```python
from build123d import *

# Parameters (mm, degrees)
SKETCH1_R           = 10
BOSS_EXTRUDE1_DEPTH = 10
FILLET1_R           = 1.5
SKETCH2_R           = 3
CUT_EXTRUDE1_DEPTH  = 8
CHAMFER1_SIZE       = 1


with BuildPart() as part:
    # Sketch1 → Boss-Extrude1 (new body)
    with BuildSketch(Plane.XY):
        Circle(SKETCH1_R)
    extrude(amount=BOSS_EXTRUDE1_DEPTH)

    # Fillet1
    fillet1_edges = [part.edges().sort_by_distance(p)[0] for p in [
        (-10, 0, 0),
        (-10, 0, 10),
    ]]
    fillet(fillet1_edges, radius=FILLET1_R)

    # Sketch2 → Cut-Extrude1 (cut)
    with BuildSketch(Plane(origin=(0, 0, 0), x_dir=(-1, 0, 0), z_dir=(0, 0, -1))):
        Circle(SKETCH2_R)
    extrude(amount=-CUT_EXTRUDE1_DEPTH, mode=Mode.SUBTRACT)

    # Chamfer1
    chamfer1_edges = [part.edges().sort_by_distance(p)[0] for p in [
        (3, 0, 0),
    ]]
    chamfer(chamfer1_edges, length=CHAMFER1_SIZE)

    # Sketch3 → Cut-Revolve2 (revolve, cut)
    with BuildSketch(Plane(origin=(0, 0, 0), x_dir=(0, 0, -1), z_dir=(1, 0, 0))):
        with BuildLine():
            Line((-19, -5), (-9, -5))
            ThreePointArc((-9, -5), (-14, -10), (-19, -5))
        make_face()
    revolve(axis=Axis((0, -5, 19), (0, 0, -1)), mode=Mode.SUBTRACT)


solid = part.part
```
For this review, take the finished solid that the model builds, in its own axes (mm). A direction names the side the tool comes from. Coordinates: 2 decimals unless noted, no trailing zeros. Order: outer loops, then holes, each group sorted by start corner. A loop starts at its lowest first (then second) coordinate and runs counter-clockwise, first axis right, second up. Notation, with made-up numbers: (55, 3) -> (98, 3) arc R10 cw to (98, 8) -> close; hole circle Ø2 at (1, 10). An arc over 180 degrees is marked (long way). Use CSV: the item, a comma, the result in double quotes. Start each with the question number.
Item 1: Draft analysis for pull direction Y (two halves, no side actions). For faces 3 (the face through (4, -2, 0)), 4 (the face through (3, 0, 4)), 5 (the face through (-2.17, -9.76, 4.95)), state which applies: pulls with the +Y half, pulls with the -Y half, needs draft (parallel to the pull), parting line crosses it, or undercut.
Item 2: Insertion check: pin 1 (5 mm diameter, centred on y = -4.5, z = 4.5, fed in from -X); pin 2 (4 mm diameter, centred on y = 7, z = 6, fed in from +X); pin 3 (6 mm diameter, centred on x = 0, y = -4.5, fed in from +Z); pin 4 (1 mm diameter, centred on y = 4.5, z = 5, fed in from +X). Each pin has a flat end and moves straight along its axis. Give the tip position at first contact, or say it passes through.
Item 3: For faces 1 (the face through (0, 0, 10)), 2 (the face through (0, 0, 8)), list the 3-axis set-ups (+Z, -Z, +X, -X, +Y, -Y) from which the entire face can be reached by the end or side of a thin tool; tool diameter is ignored.
Item 4: We need section B-B, the plane x = 0. Give the boundary of the cut face in (y, z), then the cut area to 3 significant figures.
Item 5: We need section A-A, the plane y = 0. Give the boundary of the cut face in (x, z), then the cut area to 3 significant figures.
Item 6: Wall thickness on probe 1 along Y at (x, z) = (0, 4.25); probe 2 along X at (y, z) = (3, 0.5); probe 3 along Y at (x, z) = (2, 1.5): over which ranges is each line inside the solid? List them lowest first.
Item 7: We need section C-C, the plane z = 3. Give the boundary of the cut face in (x, y), then the cut area to 3 significant figures.
Derived:
1,face 3,"needs draft"
1,face 4,"undercut"
1,face 5,"parting line crosses it"
2,pin 1,"stops at x = -9.8"
2,pin 2,"stops at x = 8.66"
2,pin 3,"stops at z = 10"
2,pin 4,"stops at x = 9.17"
3,face 1,"+Z, +X, -X, +Y, -Y"
3,face 2,"-Z"
4,outline,"(-10, 1.5) arc R1.5 ccw to (-8.5, 0) -> (-4, 0) -> (-3, 1) -> (-3, 8) -> (3, 8) -> (3, 1) -> (4, 0) -> (8.5, 0) arc R1.5 ccw to (10, 1.5) -> (10, 8.5) arc R1.5 ccw to (8.5, 10) -> (-2, 10) arc R5 cw to (-8, 10) -> (-8.5, 10) arc R1.5 ccw to (-10, 8.5) -> close"
4,area,"145 mm^2"
5,outline,"(-10, 1.5) arc R1.5 ccw to (-8.5, 0) -> (-4, 0) -> (-3, 1) -> (-3, 8) -> (3, 8) -> (3, 1) -> (4, 0) -> (8.5, 0) arc R1.5 ccw to (10, 1.5) -> (10, 8.5) arc R1.5 ccw to (8.5, 10) -> (-8.5, 10) arc R1.5 ccw to (-10, 8.5) -> close"
5,area,"149 mm^2"
6,probe 1,"y = -10 to -3, 3 to 10"
6,probe 2,"x = -9.14 to -1.8, 1.8 to 9.14"
6,probe 3,"y = -9.8 to -2.24, 2.24 to 9.8"
7,outline,"circle Ø20 at (0, 0); hole circle Ø6 at (0, 0)"
7,area,"286 mm^2"
